```python
from build123d import *

# Parameters (mm, degrees)
F1_DEPTH = 25.4
F2_R     = 1.5
F3_R     = 1.5
F4_DEPTH = 25.4
F5_R     = 2.54
F6_R     = 2.54


with BuildPart() as f1:
    # F0 (on Top) → F1 (new body)
    with BuildSketch(Plane.XY):
        Polygon((-2, -7.366), (0, -7.366), (0, 2.794), (-9.525, 2.794), (-9.525, 14.986), (0, 14.986), (0, 25.146), (-2, 25.146), (-2, 17.78), (-12.7, 17.78), (-12.7, 0), (-2, 0), align=None)
    extrude(amount=F1_DEPTH)

    # F2 (on face) + F3 (on face) → F4 (cut)
    with BuildSketch(Plane(origin=(-2, 0, 0), x_dir=(0, -1, 0), z_dir=(-1, 0, 0))):
        with Locations((4.064, 5.08)):
            Circle(F2_R)
        with Locations((4.064, 17.78)):
            Circle(F2_R)
    with BuildSketch(Plane(origin=(-2, 0, 0), x_dir=(0, -1, 0), z_dir=(-1, 0, 0))):
        with Locations((-21.59, 5.08)):
            Circle(F3_R)
        with Locations((-21.59, 17.78)):
            Circle(F3_R)
    extrude(amount=-F4_DEPTH, mode=Mode.SUBTRACT)

    # F5
    f5_edges = [f1.edges().sort_by_distance(p)[0] for p in [
        (-2, 17.78, 12.7),
        (-2, 0, 12.7),
    ]]
    fillet(f5_edges, radius=F5_R)

    # F6
    f6_edges = [f1.edges().sort_by_distance(p)[0] for p in [
        (-12.7, 0, 12.7),
        (-12.7, 17.78, 12.7),
    ]]
    fillet(f6_edges, radius=F6_R)


solid = f1.part
```
Part model, mm, in its own coordinate system. A direction names the side the tool comes from. Coordinates: 2 decimals unless noted, no trailing zeros. Write each loop counter-clockwise with the first axis right and the second up, starting at its lowest first coordinate (ties: lowest second). Pieces come first, ordered by that corner, then holes.
Item 1: Probe line 1 (Z direction, x = -1, y = 21.59); line 2 (Y direction, x = -6.75, z = 11); line 3 (Y direction, x = -1.25, z = 15.5). List the from-to ranges inside material, lowest first.
Item 2: Mould opens along Y. For faces 4 (the face through (-2.724, -0.764, 12.878)), 5 (the face through (0, 20, 13)), 6 (the face through (-9.525, 9, 13)) say: released by +Y, released by -Y, zero draft, split by the parting line, or undercut.
Item 3: Slice it at A-A (y = 21.59). Write the cut outline in (x, z).
Item 4: Pin check, flat tips, straight feed: pin 1 (1.7 mm diameter, centred on x = -6, z = 9.5, fed in from +Y); pin 2 (5 mm diameter, centred on y = 21.59, z = 17.78, fed in from -X); pin 3 (2.5 mm diameter, centred on y = -4.064, z = 5.08, fed in from -X); pin 4 (3 mm diameter, centred on x = -4, z = 6.5, fed in from -Y). Stop position of each tip, or through.
Item 5: Which spindle directions (+Z, -Z, +X, -X, +Y, -Y) get a long thin tool onto all of the face, cutting with end or side? Do faces 1 (the face through (-7, 0, 13)), 2 (the face through (-5, 14.986, 13)), 3 (the face through (-2, 23, 13)). Say none if no direction does.
Item 6: Slice it at C-C (y = 6.5). Write the cut outline in (x, z) (3 decimals), and give its area (3 significant figures).
Item 7: Slice it at B-B (z = 22.75). Write the cut outline in (x, y) (3 decimals), and give its area (3 significant figures).
Results found:
1. line 1: z = 0 to 3.58, 6.58 to 16.28, 19.28 to 25.4
1. line 2: y = 0 to 2.79, 14.99 to 17.78
1. line 3: y = -7.37 to 2.79, 14.99 to 25.15
2. face 4: released by -Y
2. face 5: zero draft
2. face 6: undercut
3. outline: (-2, 0) - (0, 0) - (0, 3.58) - (-2, 3.58) - close; (-2, 6.58) - (0, 6.58) - (0, 16.28) - (-2, 16.28) - close; (-2, 19.28) - (0, 19.28) - (0, 25.4) - (-2, 25.4) - close
4. pin 1: stops at y = 17.78
4. pin 2: stops at x = -2.31
4. pin 3: passes through
4. pin 4: stops at y = -1.03
5. face 1: +Z, -Z, -X, -Y
5. face 2: +Z, -Z, +X
5. face 3: +Z, -Z, -X, +Y
6. outline: (-12.7, 0) - (-9.525, 0) - (-9.525, 25.4) - (-12.7, 25.4) - close
6. area: 80.6 mm2
7. outline: (-12.7, 2.54) arc R2.54 ccw to (-10.16, 0) - (-4.54, 0) arc R2.54 cw to (-2, -2.54) - (-2, -7.366) - (0, -7.366) - (0, 2.794) - (-9.525, 2.794) - (-9.525, 14.986) - (0, 14.986) - (0, 25.146) - (-2, 25.146) - (-2, 20.32) arc R2.54 cw to (-4.54, 17.78) - (-10.16, 17.78) arc R2.54 ccw to (-12.7, 15.24) - close
7. area: 139 mm2
